from build123d import *

# Parameters (mm, degrees)
SKETCH_1_W          = 59.55
SKETCH_1_H          = 15
EXTRUDE_1_DEPTH     = 18.8
SKETCH_2_W          = 55.95
SKETCH_2_H          = 15
CUT_EXTRUDE_1_DEPTH = 0.8
SKETCH_4_W          = 8.2
SKETCH_4_H          = 15
CUT_EXTRUDE_2_DEPTH = 9
SKETCH_5_W          = 8.2
SKETCH_5_H          = 1.9
CUT_EXTRUDE_3_DEPTH = 15
SKETCH_6_W          = 1.5
SKETCH_6_H          = 0.75
EXTRUDE_2_DEPTH     = 5.8
SKETCH_7_R          = 2.25
CUT_EXTRUDE_4_DEPTH = 35.085783327
CUT_EXTRUDE_START   = -39.55
CUT_EXTRUDE_5_DEPTH = 39.55


with BuildPart() as part:
    # 草图1 → 拉伸1 (new body)
    with BuildSketch(Plane(origin=(0, 0, 0), x_dir=(1, 0, 0), z_dir=(0, 1, 0))):
        Rectangle(SKETCH_1_W, SKETCH_1_H)
    extrude(amount=EXTRUDE_1_DEPTH)

    # 草图2 → 切除-拉伸1 (cut)
    with BuildSketch(Plane(origin=(0, 18.8, 0), x_dir=(-1, 0, 0), z_dir=(0, 1, 0))):
        Rectangle(SKETCH_2_W, SKETCH_2_H)
    extrude(amount=-CUT_EXTRUDE_1_DEPTH, mode=Mode.SUBTRACT)

    # 草图4 → 切除-拉伸2 (cut)
    with BuildSketch(Plane(origin=(0, 18, 0), x_dir=(-1, 0, 0), z_dir=(0, 1, 0))):
        with Locations((-23.875, 0)):
            Rectangle(SKETCH_4_W, SKETCH_4_H)
        with Locations((-14.325, 0)):
            Rectangle(SKETCH_4_W, SKETCH_4_H)
        with Locations((-4.775, 0)):
            Rectangle(SKETCH_4_W, SKETCH_4_H)
        with Locations((4.775, 0)):
            Rectangle(SKETCH_4_W, SKETCH_4_H)
        with Locations((14.325, 0)):
            Rectangle(SKETCH_4_W, SKETCH_4_H)
        with Locations((23.875, 0)):
            Rectangle(SKETCH_4_W, SKETCH_4_H)
    extrude(amount=-CUT_EXTRUDE_2_DEPTH, mode=Mode.SUBTRACT)

    # 草图5 → 切除-拉伸3 (cut)
    with BuildSketch(Plane(origin=(0, 18, 0), x_dir=(-1, 0, 0), z_dir=(0, 1, 0))):
        with Locations((23.875, -6.55)):
            Rectangle(SKETCH_5_W, SKETCH_5_H)
        with Locations((23.875, 6.55)):
            Rectangle(SKETCH_5_W, SKETCH_5_H)
        with Locations((14.325, -6.55)):
            Rectangle(SKETCH_5_W, SKETCH_5_H)
        with Locations((14.325, 6.55)):
            Rectangle(SKETCH_5_W, SKETCH_5_H)
        with Locations((4.775, -6.55)):
            Rectangle(SKETCH_5_W, SKETCH_5_H)
        with Locations((4.775, 6.55)):
            Rectangle(SKETCH_5_W, SKETCH_5_H)
        with Locations((-4.775, -6.55)):
            Rectangle(SKETCH_5_W, SKETCH_5_H)
        with Locations((-4.775, 6.55)):
            Rectangle(SKETCH_5_W, SKETCH_5_H)
        with Locations((-14.325, -6.55)):
            Rectangle(SKETCH_5_W, SKETCH_5_H)
        with Locations((-14.325, 6.55)):
            Rectangle(SKETCH_5_W, SKETCH_5_H)
        with Locations((-23.875, -6.55)):
            Rectangle(SKETCH_5_W, SKETCH_5_H)
        with Locations((-23.875, 6.55)):
            Rectangle(SKETCH_5_W, SKETCH_5_H)
    extrude(amount=-CUT_EXTRUDE_3_DEPTH, mode=Mode.SUBTRACT)

    # 草图6 → 拉伸2 (add)
    with BuildSketch(Plane.XZ):
        with Locations((-4.775, 0)):
            Rectangle(SKETCH_6_W, SKETCH_6_H)
        with Locations((4.775, 0)):
            Rectangle(SKETCH_6_W, SKETCH_6_H)
        with Locations((14.325, 0)):
            Rectangle(SKETCH_6_W, SKETCH_6_H)
        with Locations((-14.325, 0)):
            Rectangle(SKETCH_6_W, SKETCH_6_H)
    extrude(amount=EXTRUDE_2_DEPTH)

    # 草图7 → 切除-拉伸4 (cut, through all)
    with BuildSketch(Plane(origin=(0, 9, 0), x_dir=(-1, 0, 0), z_dir=(0, 1, 0))):
        with Locations(Location((-23.875, 0, 0), (0, 0, 90))):
            Circle(SKETCH_7_R)
        with Locations(Location((23.875, 0, 0), (0, 0, 270))):
            Circle(SKETCH_7_R)
    extrude(amount=-CUT_EXTRUDE_4_DEPTH, mode=Mode.SUBTRACT)

    # 草图8 → 切除-拉伸5 (cut)
    with BuildSketch(Plane(origin=(19.775, 0, 0), x_dir=(0, 0, -1), z_dir=(1, 0, 0)).offset(CUT_EXTRUDE_START)):
        Polygon((7.5, 16.8), (5.4, 14.5), (7.5, 12.3), align=None)
        Polygon((-7.5, 16.8), (-7.5, 12.3), (-5.4, 14.5), align=None)
    extrude(amount=CUT_EXTRUDE_5_DEPTH, mode=Mode.SUBTRACT)


solid = part.part
Can you work these out from the model? Positions are in its coordinate system, mm. A direction names the side the tool comes from. Round coordinates to 2 decimals unless told otherwise and drop trailing zeros. Loops run counter-clockwise (first coordinate to the right, second up) from the corner with the lowest first, then second, coordinate; pieces in that order, holes last. Notation, with made-up numbers: (-16, 47) - (-10, 47) arc R22 cw to (-10, 58) - close; hole circle Ø6 at (78.25, 7). An arc over 180 degrees is marked (long way). Write item = value, one per line. Start each with the question number.
(1) For P1, Ø0.8, axis at x = 4.5, y = -2, coming from the +Z side (3 decimals); P2, Ø2, axis at x = -3, z = -7, coming from the +Y side; P3, Ø4, axis at x = 17, z = -1.5, coming from the -Y side, each with a flat end and sliding along its axis, tell me the tip position at first contact or that it passes through.
(2) If we section it at A-A (y = -1): Please give me the cut outline in (x, z) (3 decimals), and give its area (3 significant figures).
(3) If we section it at C-C (y = 13): Please give me the cut outline in (x, z) (3 decimals), and give its area (3 significant figures).
(4) For faces 4 (the face through (-14, -3, -0.375)), 5 (the face through (-24, 3, 7)), 6 (the face through (-9.559, 13.415, -6.435)), which set-ups out of +Z, -Z, +X, -X, +Y, -Y let a thin tool reach every point of the face, with its end or its side?
(5) If we section it at D-D (z = -3.5): Please give me the cut outline in (x, y) (3 decimals).
(6) If we mould it in two halves opening along X, with no side actions, what happens to faces 1 (the face through (29.775, 9, 0)), 2 (the face through (-0.009, 13.415, -6.435)), 3 (the face through (10, 17, -7.5))? For each: released by +X, released by -X, zero draft, split by the parting line, or undercut.
(7) If we section it at B-B (x = 12.5): Please give me the cut outline in (y, z).
(8) If I drill on probe 1 along X at (y, z) = (7.25, 0) (3 decimals); probe 2 along X at (y, z) = (2, -1.5) (3 decimals); probe 3 along Y at (x, z) = (-9, -4), over which ranges is the centre line in solid material (lowest first)? Write a range as [from, to].
Ans:
q1.P1 = 0.375
q1.P2 = 3
q1.P3 = 0
q2.outline = (-15.075, -0.375) - (-13.575, -0.375) - (-13.575, 0.375) - (-15.075, 0.375) - close; (-5.525, -0.375) - (-4.025, -0.375) - (-4.025, 0.375) - (-5.525, 0.375) - close; (4.025, -0.375) - (5.525, -0.375) - (5.525, 0.375) - (4.025, 0.375) - close; (13.575, -0.375) - (15.075, -0.375) - (15.075, 0.375) - (13.575, 0.375) - close
q2.area = 4.50 mm²
q3.outline = (-29.775, -7.5) - (-27.975, -7.5) - (-27.975, 7.5) - (-29.775, 7.5) - close; (-19.775, -6.832) - (-18.425, -6.832) - (-18.425, 6.832) - (-19.775, 6.832) - close; (-10.225, -6.832) - (-8.875, -6.832) - (-8.875, 6.832) - (-10.225, 6.832) - close; (-0.675, -6.832) - (0.675, -6.832) - (0.675, 6.832) - (-0.675, 6.832) - close; (8.875, -6.832) - (10.225, -6.832) - (10.225, 6.832) - (8.875, 6.832) - close; (18.425, -6.832) - (19.775, -6.832) - (19.775, 6.832) - (18.425, 6.832) - close; (27.975, -7.5) - (29.775, -7.5) - (29.775, 7.5) - (27.975, 7.5) - close
q3.area = 146 mm²
q4.face_4 = -Z, +X, -X, -Y
q4.face_5 = +Z, +Y
q4.face_6 = -Z
q5.outline = (-29.775, 0) - (29.775, 0) - (29.775, 18.8) - (27.975, 18.8) - (27.975, 9) - (19.775, 9) - (19.775, 18) - (18.425, 18) - (18.425, 9) - (10.225, 9) - (10.225, 18) - (8.875, 18) - (8.875, 9) - (0.675, 9) - (0.675, 18) - (-0.675, 18) - (-0.675, 9) - (-8.875, 9) - (-8.875, 18) - (-10.225, 18) - (-10.225, 9) - (-18.425, 9) - (-18.425, 18) - (-19.775, 18) - (-19.775, 9) - (-27.975, 9) - (-27.975, 18.8) - (-29.775, 18.8) - close
q6.face_1 = released by +X
q6.face_2 = undercut
q6.face_3 = zero draft
q7.outline = (0, -7.5) - (3, -7.5) - (3, -5.6) - (9, -5.6) - (9, 5.6) - (3, 5.6) - (3, 7.5) - (0, 7.5) - close
q8.probe_1 = [-29.775, -26.125], [-21.625, 21.625], [26.125, 29.775]
q8.probe_2 = [-29.775, -25.552], [-22.198, 22.198], [25.552, 29.775]
q8.probe_3 = [0, 18]
